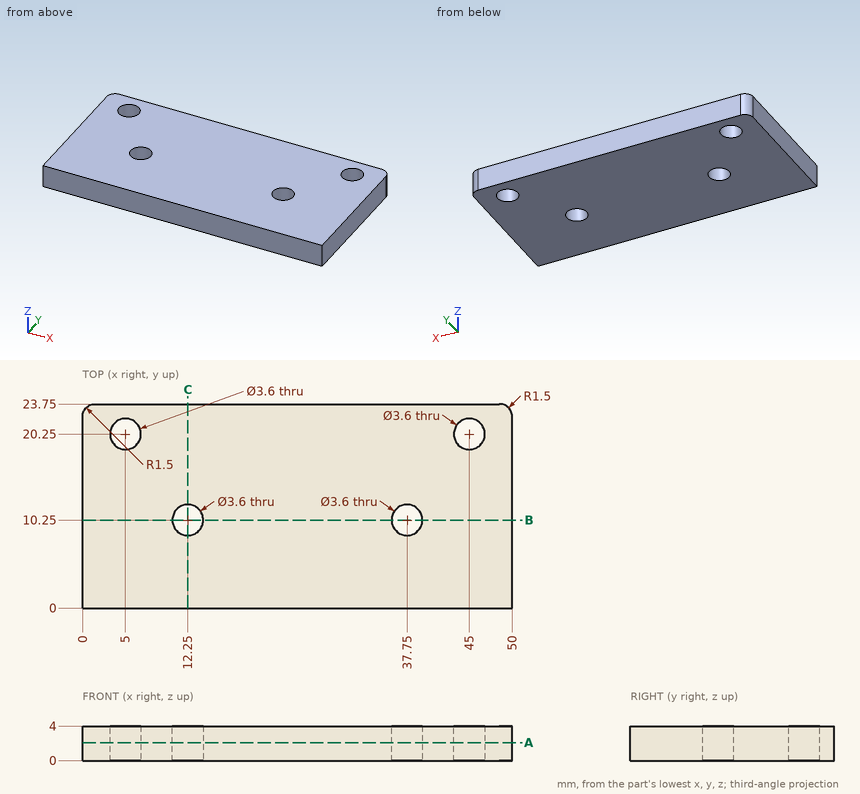
Print and shaded views of the part. All mm, measured from the part's lowest x, y and z. Give positions to 0.01 mm unless a question says otherwise; leave off trailing zeros. Loops run counter-clockwise (first coordinate to the right, second up) from the corner with the lowest first, then second, coordinate; pieces in that order, holes last.
1) Saw through at C-C (x = 12.25). Write the cut outline in (y, z).
2) Saw through at B-B (y = 10.25). Write the cut outline in (x, z), plus the area to 3 significant figures.
3) Wall check: line 1 (Y direction, x = 37.75, z = 1.8); line 2 (X direction, y = 10.5, z = 1.75); line 3 (X direction, y = 11.25, z = 0.85). Give the ranges that are in metal, low to high.
4) Saw through at A-A (z = 2.1). Write the cut outline in (x, y).
Answer block:
1. outline: (0, 0) - (8.45, 0) - (8.45, 4) - (0, 4) - close; (12.05, 0) - (23.75, 0) - (23.75, 4) - (12.05, 4) - close
2. outline: (0, 0) - (10.45, 0) - (10.45, 4) - (0, 4) - close; (14.05, 0) - (35.95, 0) - (35.95, 4) - (14.05, 4) - close; (39.55, 0) - (50, 0) - (50, 4) - (39.55, 4) - close
2. area: 171 mm2
3. line 1: y = 0 to 8.45, 12.05 to 23.75
3. line 2: x = 0 to 10.47, 14.03 to 35.97, 39.53 to 50
3. line 3: x = 0 to 10.75, 13.75 to 36.25, 39.25 to 50
4. outline: (0, 0) - (50, 0) - (50, 22.25) arc R1.5 ccw to (48.5, 23.75) - (1.5, 23.75) arc R1.5 ccw to (0, 22.25) - close; hole circle Ø3.6 at (5, 20.25); hole circle Ø3.6 at (12.25, 10.25); hole circle Ø3.6 at (37.75, 10.25); hole circle Ø3.6 at (45, 20.25)
